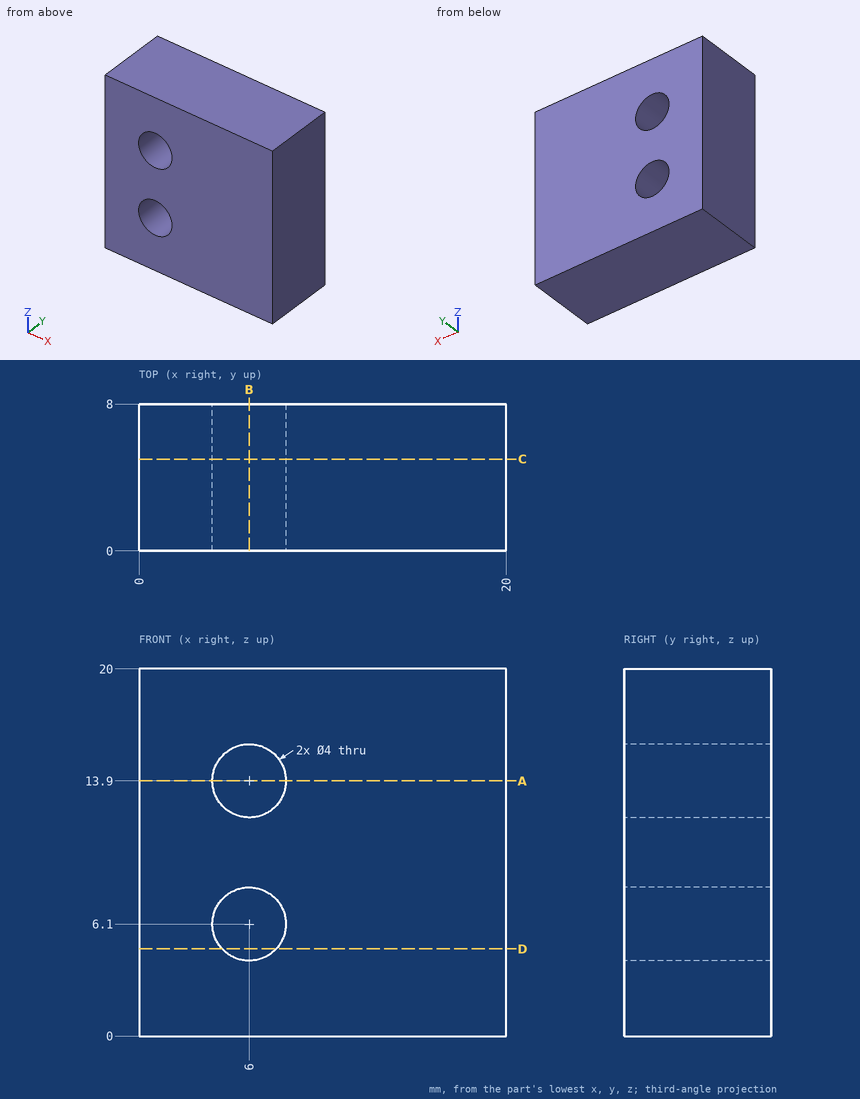
Geometry: see drawing. Coordinates: mm, zero at the bounding-box minimum. Give positions to 0.01 mm unless a question says otherwise; leave off trailing zeros. Write each loop counter-clockwise with the first axis right and the second up, starting at its lowest first coordinate (ties: lowest second). Pieces come first, ordered by that corner, then holes. Notation, with made-up numbers: M 77,62 L 131,62 A22 ccw 131,71 Z; hole C -35,16 d9. An arc over 180 degrees is marked long. Answer in a Markdown table with one row per item. Add a question column.
(1) Section C-C on y = 5. Return loops of the section in (x, z), and give its area (3 significant figures).
(2) Ray query, line 1 (Z direction, x = 6, y = 5); line 2 (Z direction, x = 6.75, y = 5); line 3 (X direction, y = 3.5, z = 7.75). Return the intervals inside material, ascending.
(3) Section D-D on z = 4.75. Return loops of the section in (x, y).
(4) Section B-B on x = 6. Return loops of the section in (y, z).
(5) Section A-A on z = 13.9. Return loops of the section in (x, y), and give its area (3 significant figures).
Result set:
| question | item | result |
|---|---|---|
| 1 | outline | M 0,0 L 20,0 L 20,20 L 0,20 Z; hole C 6,6.1 d4; hole C 6,13.9 d4 |
| 1 | area | 375 mm^2 |
| 2 | line 1 | z = 0 to 4.1, 8.1 to 11.9, 15.9 to 20 |
| 2 | line 2 | z = 0 to 4.25, 7.95 to 12.05, 15.75 to 20 |
| 2 | line 3 | x = 0 to 4.87, 7.13 to 20 |
| 3 | outline | M 0,0 L 4.52,0 L 4.52,8 L 0,8 Z; M 7.48,0 L 20,0 L 20,8 L 7.48,8 Z |
| 4 | outline | M 0,0 L 8,0 L 8,4.1 L 0,4.1 Z; M 0,8.1 L 8,8.1 L 8,11.9 L 0,11.9 Z; M 0,15.9 L 8,15.9 L 8,20 L 0,20 Z |
| 5 | outline | M 0,0 L 4,0 L 4,8 L 0,8 Z; M 8,0 L 20,0 L 20,8 L 8,8 Z |
| 5 | area | 128 mm^2 |
